Source: CAD feature listing. Evaluate the final solid. Frame: model axes, mm. Face numbers are marked on the shaded views. A direction names the side the tool comes from. Coordinates: 2 decimals unless noted, no trailing zeros. Write each loop counter-clockwise with the first axis right and the second up, starting at its lowest first coordinate (ties: lowest second). Pieces come first, ordered by that corner, then holes. Notation, with made-up numbers: M 57.25,-23.75 L 101.25,-23.75 A16 cw 101.25,-18.75 Z; hole C -16.5,46.25 d9. An arc over 180 degrees is marked long. One line per item, written item: value. Start each with the question number.
Item 1: Mould query, pull axis X, two halves, no side actions, for the marked faces 1, 2 and 3. Classes: released by +X, released by -X, zero draft, split by the parting line, or undercut.
Item 2: Cut plane A-A, the plane z = -3. Output: boundary loops of the cut face in (x, y), then the cut area to 3 significant figures.
Item 3: Cut plane B-B, the plane x = 3. Output: boundary loops of the cut face in (y, z), then the cut area to 3 significant figures.
Item 4: Cut plane D-D, the plane z = 2. Output: boundary loops of the cut face in (x, y), then the cut area to 3 significant figures.
Item 5: Set-up query: the marked faces 4 and 5. Return all of +Z, -Z, +X, -X, +Y, -Y with unobstructed straight access to the full face (end or side cutting, diameter ignored); none if empty.
Item 6: Ray query, L1, parallel to Z at x = -3, y = -0.6; L2, parallel to Z at x = 3, y = -1.5; L3, parallel to X at y = -0.05, z = 2. Return the intervals inside material, ascending. Write a range as from..to.
Item 7: Pin query (flat end, axial travel): P1, Ø2, axis at x = 2.5, y = 2, coming from the +Z side; P2, Ø1, axis at x = -4.5, y = -0.5, coming from the +Z side; P3, Ø5, axis at x = -3, z = -3, coming from the +Y side. Return the tip coordinate at first contact, or that it passes through.
Item 8: Cut plane C-C, the plane x = -2.25. Output: boundary loops of the cut face in (y, z), then the cut area to 3 significant figures.
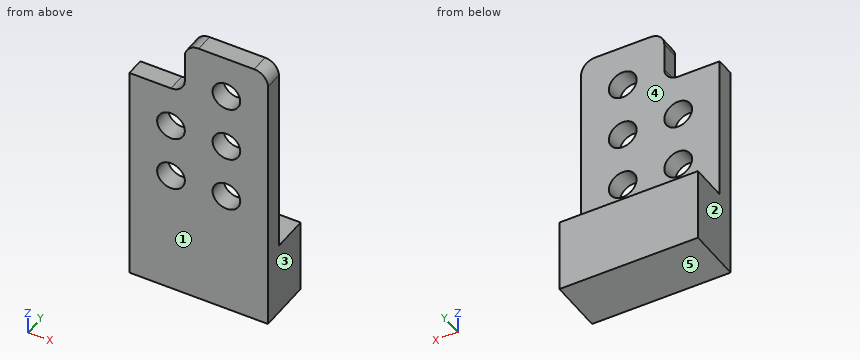
```python
from build123d import *

# Parameters (mm, degrees)
F0_W      = 15
F0_H      = 15
F1_DEPTH  = 2
F2_R      = 1.5
F3_DEPTH  = 25
F4_W      = 9
F4_H      = 2
F5_DEPTH  = 6
F6_R      = 1.5
F7_DEPTH  = 25
F8_R      = 1.5
F9_W      = 15
F9_H      = 2
F10_DEPTH = 1
F11_W     = 15
F11_H     = 6
F12_DEPTH = 8


with BuildPart() as f1:
    # F0 (on Front) → F1 (new body)
    with BuildSketch(Plane.XZ):
        Rectangle(F0_W, F0_H)
    extrude(amount=F1_DEPTH)

    # F2 (on face) → F3 (cut)
    with BuildSketch(Plane.XZ.offset(2)):
        with Locations((3, 3)):
            Circle(F2_R)
        with Locations((-3, 3)):
            Circle(F2_R)
        with Locations((-3, -3)):
            Circle(F2_R)
        with Locations((3, -3)):
            Circle(F2_R)
    extrude(amount=-F3_DEPTH, mode=Mode.SUBTRACT)

    # F4 (on face) → F5 (join)
    with BuildSketch(Plane.XY.offset(7.5)):
        with Locations((3, -1)):
            Rectangle(F4_W, F4_H)
    extrude(amount=F5_DEPTH)

    # F6 (on face) → F7 (cut)
    with BuildSketch(Plane.XZ.offset(2)):
        with Locations((3, 9)):
            Circle(F6_R)
    extrude(amount=-F7_DEPTH, mode=Mode.SUBTRACT)

    # F8
    f8_edges = [f1.edges().sort_by_distance(p)[0] for p in [
        (7.5, -1, 13.5),
        (-1.5, -1, 13.5),
        (-1.5, -1, 7.5),
    ]]
    fillet(f8_edges, radius=F8_R)

    # F9 (on face) → F10 (join)
    with BuildSketch(Plane(origin=(0, 0, -7.5), x_dir=(1, 0, 0), z_dir=(0, 0, -1))):
        with Locations((0, 1)):
            Rectangle(F9_W, F9_H)
    extrude(amount=F10_DEPTH)

    # F11 (on face) → F12 (join)
    with BuildSketch(Plane(origin=(0, 0, -8.5), x_dir=(1, 0, 0), z_dir=(0, 0, -1))):
        with Locations((0, -1)):
            Rectangle(F11_W, F11_H)
    extrude(amount=F12_DEPTH)


solid = f1.part
```
From the geometry:
1. face 1: zero draft
1. face 2: released by -X
1. face 3: released by +X
2. outline: M -7.5,-2 L -4.5,-2 L -4.5,0 L -7.5,0 Z; M -1.5,-2 L 1.5,-2 L 1.5,0 L -1.5,0 Z; M 4.5,-2 L 7.5,-2 L 7.5,0 L 4.5,0 Z
2. area: 18.0 mm²
3. outline: M -2,-16.5 L 4,-16.5 L 4,-8.5 L 0,-8.5 L 0,-4.5 L -2,-4.5 Z; M -2,-1.5 L 0,-1.5 L 0,1.5 L -2,1.5 Z; M -2,4.5 L 0,4.5 L 0,7.5 L -2,7.5 Z; M -2,10.5 L 0,10.5 L 0,13.5 L -2,13.5 Z
3. area: 74.0 mm²
4. outline: M -7.5,-2 L -4.12,-2 L -4.12,0 L -7.5,0 Z; M -1.88,-2 L 1.88,-2 L 1.88,0 L -1.88,0 Z; M 4.12,-2 L 7.5,-2 L 7.5,0 L 4.12,0 Z
4. area: 21.1 mm²
5. face 4: +Z, +X, -X, +Y
5. face 5: -Z, +X, -X, +Y, -Y
6. L1: z = -16.5..-4.5, -1.5..1.5, 4.5..7.5
6. L2: z = -16.5..-4.5, -1.5..1.5, 4.5..7.5, 10.5..13.5
6. L3: x = -7.5..-4.12, -1.88..1.88, 4.12..7.5
7. P1: stops at z = -8.5
7. P2: stops at z = 7.5
7. P3: stops at y = 0
8. outline: M -2,-16.5 L 4,-16.5 L 4,-8.5 L 0,-8.5 L 0,-4.3 L -2,-4.3 Z; M -2,-1.7 L 0,-1.7 L 0,1.7 L -2,1.7 Z; M -2,4.3 L 0,4.3 L 0,7.7 L -2,7.7 Z
8. area: 70.0 mm²
